The model under review builds one solid part; all positions refer to its coordinate system, in mm. Face numbers are marked on the shaded views. A direction names the side the tool comes from. Give positions to 0.01 mm unless a question says otherwise; leave off trailing zeros. Loops run counter-clockwise (first coordinate to the right, second up) from the corner with the lowest first, then second, coordinate; pieces in that order, holes last. Notation, with made-up numbers: M 3,44 L 51,44 A18 cw 51,59 Z; hole C 88,45 d10. An arc over 180 degrees is marked long. Write item = value, one per line. Start each with the question number.
1. We need section C-C on x = 72.5. Give the boundary of the cut face in (y, z), then the cut area to 3 significant figures.
2. Wall thickness on line 1 along Y through (x, z) = (124, 0); line 2 along Y through (x, z) = (112, 0); line 3 along X through (y, z) = (11, -12): over which ranges is each line inside the solid? List them lowest first. Write a range as from..to.
3. We need section A-A on x = 23. Give the boundary of the cut face in (y, z).
4. We need section B-B on x = 116.5. Give the boundary of the cut face in (y, z), then the cut area to 3 significant figures.
5. For pin 1 (2 mm diameter, centred on y = -12.5, z = 27.5, fed in from -X); pin 2 (0.5 mm diameter, centred on x = 39.5, y = -11.5, fed in from -Z); pin 3 (1 mm diameter, centred on x = 98.5, z = -12, fed in from -Y), all flat-tipped, find the tip position at first contact; note any pin that passes through.
6. Draft analysis for pull direction Z (two halves, no side actions). For the marked faces 4, 5 and 6, state which applies: pulls with the +Z half, pulls with the -Z half, needs draft (parallel to the pull), parting line crosses it, or undercut.
7. For the marked faces 1, 2 and 3, list the 3-axis set-ups (+Z, -Z, +X, -X, +Y, -Y) from which the entire face can be reached by the end or side of a thin tool; tool diameter is ignored.
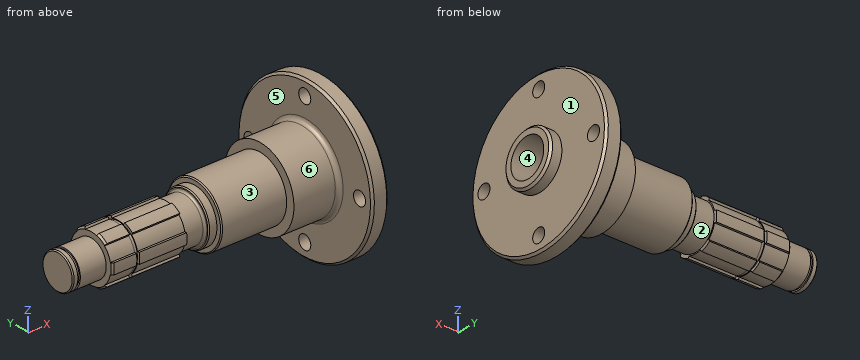
from build123d import *

# Parameters (mm, degrees)
ESQUISSE1_W                  = 135
ESQUISSE1_H                  = 37.5
D_GAGEMENT_M61_D             = 6.6
R_P_TITION_CIRCULAIRE1_COUNT = 4
CONG_1_R                     = 2
ESQUISSE12_W                 = 1.4
ESQUISSE12_H                 = 1.27
ESQUISSE7_R                  = 13.345253716
ENL_V_MAT_EXTRU_1_DEPTH      = 36
ESQUISSE8_W                  = 1.2
ESQUISSE8_H                  = 0.65
CHANFREIN1_SIZE              = 0.8
CHANFREIN2_SIZE              = 0.5
CONG_2_R                     = 1
CHANFREIN3_SIZE              = 0.5
CHANFREIN4_SIZE              = 1
CHANFREIN5_SIZE              = 1
CHANFREIN6_SIZE              = 0.5


with BuildPart() as part:
    # Esquisse1 → Révolution1 (revolve)
    with BuildSketch(Plane.XY, mode=Mode.PRIVATE) as r_volution1_sk:
        with Locations((67.5, 18.75)):
            Rectangle(ESQUISSE1_W, ESQUISSE1_H)
    revolve(r_volution1_sk.sketch.rotate(Axis((-44.672408566, 0, 0), (1, 0, 0)), 90), axis=Axis((-44.672408566, 0, 0), (1, 0, 0)))  # turned: the seam where the file's is

    # Esquisse2 → Enlèvement de matière-Révolution1 (revolve, cut)
    with BuildSketch(Plane.XY, mode=Mode.PRIVATE) as enl_vement_de_mati_re_r_volution1_sk:
        Polygon((0, 0), (0, 37.5), (135, 37.5), (135, 0), (134, 0), (134, 12.7), (128.5, 12.7), (128.5, 37), (120.5, 37), (120.5, 19), (98.5, 19), (98.5, 15), (53, 15), (53, 12.02), (17, 12.02), (17, 8.5), (1, 8.5), (1, 0), align=None)
    revolve(enl_vement_de_mati_re_r_volution1_sk.sketch.rotate(Axis((-11.79532693, 0, 0), (1, 0, 0)), 90), axis=Axis((-11.79532693, 0, 0), (1, 0, 0)), mode=Mode.SUBTRACT)  # turned: the seam where the file's is

    # Dégagement M61 (through all)
    with Locations(Plane(origin=(128.5, 0, 0), x_dir=(0, 0, -1), z_dir=(1, 0, 0))):
        with Locations((0, 30)):
            d_gagement_m61 = Hole(D_GAGEMENT_M61_D / 2)

    # Répétition circulaire1: Dégagement M61 ×4 about axis
    r_p_tition_circulaire1_axis = Axis((0, 0, 0), (1, 0, 0))
    for i in range(1, R_P_TITION_CIRCULAIRE1_COUNT):
        add(d_gagement_m61.rotate(r_p_tition_circulaire1_axis, i * 360 / R_P_TITION_CIRCULAIRE1_COUNT), mode=Mode.SUBTRACT)

    # Congé1
    cong_1_edges = [part.edges().sort_by_distance(p)[0] for p in [
        (120.5, 0, -19),
    ]]
    fillet(cong_1_edges, radius=CONG_1_R)

    # Esquisse12 → Enlèvement de matière-Révolution6 (revolve, cut)
    with BuildSketch(Plane.XY, mode=Mode.PRIVATE) as enl_vement_de_mati_re_r_volution6_sk:
        with Locations((29.4, 11.385)):
            Rectangle(ESQUISSE12_W, ESQUISSE12_H)
    revolve(enl_vement_de_mati_re_r_volution6_sk.sketch.rotate(Axis((0, 0, 0), (-1, 0, 0)), 270), axis=Axis((0, 0, 0), (-1, 0, 0)), mode=Mode.SUBTRACT)  # turned: the seam where the file's is

    # Esquisse7 → Enlèv. mat.-Extru.1 (cut)
    with BuildSketch(Plane.ZY.offset(-17)):
        Circle(ESQUISSE7_R)
        with BuildLine():
            Line((11.43198409, 3.713507746), (10.571447044, 3.216676451))
            ThreePointArc((10.571447044, 3.216676451), (11.05, 0), (10.571447044, -3.216676451))
            Line((10.571447044, -3.216676451), (11.43198409, -3.713507746))
            ThreePointArc((11.43198409, -3.713507746), (10.409625353, -6.01), (8.93198409, -8.043634764))
            Line((8.93198409, -8.043634764), (8.071447044, -7.54680347))
            ThreePointArc((8.071447044, -7.54680347), (5.525, -9.569580712), (2.5, -10.763479921))
            Line((2.5, -10.763479921), (2.5, -11.75714251))
            ThreePointArc((2.5, -11.75714251), (0, -12.02), (-2.5, -11.75714251))
            Line((-2.5, -11.75714251), (-2.5, -10.763479921))
            ThreePointArc((-2.5, -10.763479921), (-5.525, -9.569580712), (-8.071447044, -7.54680347))
            Line((-8.071447044, -7.54680347), (-8.93198409, -8.043634764))
            ThreePointArc((-8.93198409, -8.043634764), (-10.409625353, -6.01), (-11.43198409, -3.713507746))
            Line((-11.43198409, -3.713507746), (-10.571447044, -3.216676451))
            ThreePointArc((-10.571447044, -3.216676451), (-11.05, 0), (-10.571447044, 3.216676451))
            Line((-10.571447044, 3.216676451), (-11.43198409, 3.713507746))
            ThreePointArc((-11.43198409, 3.713507746), (-10.409625353, 6.01), (-8.93198409, 8.043634764))
            Line((-8.93198409, 8.043634764), (-8.071447044, 7.54680347))
            ThreePointArc((-8.071447044, 7.54680347), (-5.525, 9.569580712), (-2.5, 10.763479921))
            Line((-2.5, 10.763479921), (-2.5, 11.75714251))
            ThreePointArc((-2.5, 11.75714251), (0, 12.02), (2.5, 11.75714251))
            Line((2.5, 11.75714251), (2.5, 10.763479921))
            ThreePointArc((2.5, 10.763479921), (5.525, 9.569580712), (8.071447044, 7.54680347))
            Line((8.071447044, 7.54680347), (8.93198409, 8.043634764))
            ThreePointArc((8.93198409, 8.043634764), (10.409625353, 6.01), (11.43198409, 3.713507746))
        make_face(mode=Mode.SUBTRACT)
    extrude(amount=-ENL_V_MAT_EXTRU_1_DEPTH, mode=Mode.SUBTRACT)

    # Esquisse8 → Enlèvement de matière-Révolution3 (revolve, cut)
    with BuildSketch(Plane.XY, mode=Mode.PRIVATE) as enl_vement_de_mati_re_r_volution3_sk:
        with Locations((3.9, 8.175)):
            Rectangle(ESQUISSE8_W, ESQUISSE8_H)
    revolve(enl_vement_de_mati_re_r_volution3_sk.sketch.rotate(Axis((-5.65, 0, 0), (1, 0, 0)), 90), axis=Axis((-5.65, 0, 0), (1, 0, 0)), mode=Mode.SUBTRACT)  # turned: the seam where the file's is

    # Chanfrein1
    chanfrein1_edges = [part.edges().sort_by_distance(p)[0] for p in [
        (17, 6.01, 10.409625353),
        (17, 12.02, 0),
        (17, 6.01, -10.409625353),
        (17, -6.01, -10.409625353),
        (17, -12.02, 0),
        (17, -6.01, 10.409625353),
    ]]
    chamfer(chanfrein1_edges, length=CHANFREIN1_SIZE)

    # Esquisse9 → Enlèvement de matière-Révolution4 (revolve, cut)
    with BuildSketch(Plane.XY, mode=Mode.PRIVATE) as enl_vement_de_mati_re_r_volution4_sk:
        Polygon((53, 15), (67, 15), (67, 12.5), (63, 12.5), (63, 10.5), (53, 10.5), align=None)
    revolve(enl_vement_de_mati_re_r_volution4_sk.sketch.rotate(Axis((-5.65, 0, 0), (1, 0, 0)), 90), axis=Axis((-5.65, 0, 0), (1, 0, 0)), mode=Mode.SUBTRACT)  # turned: the seam where the file's is

    # Chanfrein2
    chanfrein2_edges = [part.edges().sort_by_distance(p)[0] for p in [
        (67, 0, -15),
    ]]
    chamfer(chanfrein2_edges, length=CHANFREIN2_SIZE)

    # Congé2
    cong_2_edges = [part.edges().sort_by_distance(p)[0] for p in [
        (63, 0, -10.5),
    ]]
    fillet(cong_2_edges, radius=CONG_2_R)

    # Chanfrein3
    chanfrein3_edges = [part.edges().sort_by_distance(p)[0] for p in [
        (1, 0, -8.5),
    ]]
    chamfer(chanfrein3_edges, length=CHANFREIN3_SIZE)

    # Chanfrein4
    chanfrein4_edges = [part.edges().sort_by_distance(p)[0] for p in [
        (128.5, 0, -37),
        (120.5, 0, -37),
    ]]
    chamfer(chanfrein4_edges, length=CHANFREIN4_SIZE)

    # Chanfrein5
    chanfrein5_edges = [part.edges().sort_by_distance(p)[0] for p in [
        (134, 0, -12.7),
    ]]
    chamfer(chanfrein5_edges, length=CHANFREIN5_SIZE)

    # Chanfrein6
    chanfrein6_edges = [part.edges().sort_by_distance(p)[0] for p in [
        (63, 0, -12.5),
    ]]
    chamfer(chanfrein6_edges, length=CHANFREIN6_SIZE)

    # Esquisse13 → Enlèvement de matière-Révolution7 (revolve, cut)
    with BuildSketch(Plane.XY, mode=Mode.PRIVATE) as enl_vement_de_mati_re_r_volution7_sk:
        Polygon((134, 9), (74.196152423, 9), (69, 0), (134, 0), align=None)
    revolve(enl_vement_de_mati_re_r_volution7_sk.sketch.rotate(Axis((-5.65, 0, 0), (1, 0, 0)), 90), axis=Axis((-5.65, 0, 0), (1, 0, 0)), mode=Mode.SUBTRACT)  # turned: the seam where the file's is


solid = part.part
Final values:
q1.outline = C 0,0 d30; hole C 0,0 d12.12
q1.area = 591 mm²
q2.line_1 = -37..-33.3, -26.7..-9, 9..26.7, 33.3..37
q2.line_2 = -19..-9, 9..19
q2.line_3 = 98.5..128.5
q3.outline = M -11.76,-2.5 L -10.76,-2.5 A11.05 ccw -7.55,-8.07 L -8.04,-8.93 A12.02 ccw -3.71,-11.43 L -3.22,-10.57 A11.05 ccw 3.22,-10.57 L 3.71,-11.43 A12.02 ccw 8.04,-8.93 L 7.55,-8.07 A11.05 ccw 10.76,-2.5 L 11.76,-2.5 A12.02 ccw 11.76,2.5 L 10.76,2.5 A11.05 ccw 7.55,8.07 L 8.04,8.93 A12.02 ccw 3.71,11.43 L 3.22,10.57 A11.05 ccw -3.22,10.57 L -3.71,11.43 A12.02 ccw -8.04,8.93 L -7.55,8.07 A11.05 ccw -10.76,2.5 L -11.76,2.5 A12.02 ccw Z
q4.outline = C 0,0 d38; hole C 0,0 d18
q4.area = 880 mm²
q5.pin_1 = 120.5
q5.pin_2 = -2.5
q5.pin_3 = -15.12
q6.face_4 = undercut
q6.face_5 = needs draft
q6.face_6 = parting line crosses it
q7.face_1 = +X
q7.face_2 = none
q7.face_3 = -X
